```python
from build123d import *

# Parameters (mm, degrees)
BOSS_EXTRUDE1_DEPTH = 2.5
CUT_EXTRUDE1_DEPTH  = 10.5
FILLET1_R           = 0.25
CUT_EXTRUDE2_DEPTH  = 5.25
BOSS_EXTRUDE2_DEPTH = 0.5
CHAMFER1_SIZE       = 0.6
CHAMFER2_SIZE       = 0.4


with BuildPart() as part:
    # Sketch1 → Boss-Extrude1 (new body)
    with BuildSketch(Plane.XY):
        with BuildLine():
            Line((-2.75, -4), (-2.75, 4.05))
            ThreePointArc((-2.75, 4.05), (-2.544974747, 4.544974747), (-2.05, 4.75))
            Line((-2.05, 4.75), (2.05, 4.75))
            ThreePointArc((2.05, 4.75), (2.544974747, 4.544974747), (2.75, 4.05))
            Line((2.75, 4.05), (2.75, -4))
            Line((2.75, -4), (2.25, -4))
            Line((2.25, -4), (2.25, 4.05))
            ThreePointArc((2.25, 4.05), (2.191421356, 4.191421356), (2.05, 4.25))
            Line((2.05, 4.25), (-2.05, 4.25))
            ThreePointArc((-2.05, 4.25), (-2.191421356, 4.191421356), (-2.25, 4.05))
            Line((-2.25, 4.05), (-2.25, -4))
            Line((-2.25, -4), (-2.75, -4))
        make_face()
    extrude(amount=BOSS_EXTRUDE1_DEPTH)

    # Sketch2 → Cut-Extrude1 (cut)
    with BuildSketch(Plane(origin=(0, 4.75, 0), x_dir=(1, 0, 0), z_dir=(0, 1, 0))):
        with BuildLine():
            Line((-2.05, 0), (-1.725962279, -0.216025147))
            ThreePointArc((-1.725962279, -0.216025147), (-1.593504255, -0.278546013), (-1.448612181, -0.3))
            Line((-1.448612181, -0.3), (1.448612181, -0.3))
            ThreePointArc((1.448612181, -0.3), (1.593504255, -0.278546013), (1.725962279, -0.216025147))
            Line((1.725962279, -0.216025147), (2.05, 0))
            Line((2.05, 0), (2.05, 0.547519398))
            Line((2.05, 0.547519398), (-2.05, 0.547519398))
            Line((-2.05, 0.547519398), (-2.05, 0))
        make_face()
        with BuildLine():
            Line((-2.75, -2.5), (-2.345189488, -2.5))
            ThreePointArc((-2.345189488, -2.5), (-2.090994028, -2.430563198), (-1.907400646, -2.241538671))
            Line((-1.907400646, -2.241538671), (-1.321299677, -1.179230664))
            ThreePointArc((-1.321299677, -1.179230664), (-1.229502986, -1.084718401), (-1.102405256, -1.05))
            Line((-1.102405256, -1.05), (1.084290526, -1.05))
            ThreePointArc((1.084290526, -1.05), (1.222412736, -1.091619926), (1.314545856, -1.202621958))
            Line((1.314545856, -1.202621958), (1.734132573, -2.194756083))
            ThreePointArc((1.734132573, -2.194756083), (1.918398814, -2.416760148), (2.194643233, -2.5))
            Line((2.194643233, -2.5), (2.75, -2.5))
            Line((2.75, -2.5), (2.75, -3.056093585))
            Line((2.75, -3.056093585), (-2.75, -3.056093585))
            Line((-2.75, -3.056093585), (-2.75, -2.5))
        make_face()
    extrude(amount=-CUT_EXTRUDE1_DEPTH, mode=Mode.SUBTRACT)

    # Fillet1
    fillet1_edges = [part.edges().sort_by_distance(p)[0] for p in [
        (-2.05, 4.5, 0),
        (2.05, 4.5, 0),
    ]]
    fillet(fillet1_edges, radius=FILLET1_R)

    # Sketch3 → Cut-Extrude2 (cut, symmetric)
    with BuildSketch(Plane(origin=(0, 0, 0), x_dir=(0, 0, -1), z_dir=(1, 0, 0))):
        Polygon((0, 0.25), (-0.5, -0.35), (-0.5, -4.396314828), (0.876390697, -4.396314828), (0.876390697, 0.25), align=None)
        Polygon((-2.5, 0.25), (-2, -0.35), (-2, -4.896314828), (-3.070294312, -4.896314828), (-3.070294312, 0.25), align=None)
        with BuildLine():
            Line((-0.75, 3.024565065), (-0.75, 1.024565065))
            ThreePointArc((-0.75, 1.024565065), (-1.25, 0.524565065), (-1.75, 1.024565065))
            Line((-1.75, 1.024565065), (-1.75, 3.024565065))
            ThreePointArc((-1.75, 3.024565065), (-1.25, 3.524565065), (-0.75, 3.024565065))
        make_face()
    extrude(amount=CUT_EXTRUDE2_DEPTH, both=True, mode=Mode.SUBTRACT)

    # Sketch4 → Boss-Extrude2 (add, symmetric)
    with BuildSketch(Plane(origin=(0, 0, 0), x_dir=(0, 0, -1), z_dir=(1, 0, 0))):
        with BuildLine():
            Line((-1.05, 4.25), (-1.395169213, 3.954140675))
            ThreePointArc((-1.395169213, 3.954140675), (-1.770160684, 3.782160221), (-2.179373497, 3.834512432))
            Line((-2.179373497, 3.834512432), (-2.75, 4.079724782))
            Line((-2.75, 4.079724782), (-2.552592831, 4.539105245))
            Line((-2.552592831, 4.539105245), (-1.981966328, 4.293892895))
            ThreePointArc((-1.981966328, 4.293892895), (-1.845562057, 4.276442158), (-1.7205649, 4.333768976))
            Line((-1.7205649, 4.333768976), (-1.347308957, 4.653702641))
            ThreePointArc((-1.347308957, 4.653702641), (-1.225770907, 4.725154006), (-1.086992408, 4.75))
            Line((-1.086992408, 4.75), (-1.05, 4.75))
            Line((-1.05, 4.75), (-1.05, 4.25))
        make_face()
    extrude(amount=BOSS_EXTRUDE2_DEPTH, both=True)

    # Chamfer1
    chamfer1_edges = [part.edges().sort_by_distance(p)[0] for p in [
        (2.5, -4, 0.5),
        (-2.5, -4, 0.5),
    ]]
    chamfer(chamfer1_edges, length=CHAMFER1_SIZE)

    # Chamfer2
    chamfer2_edges = [part.edges().sort_by_distance(p)[0] for p in [
        (2.5, -4, 2),
        (-2.5, -4, 2),
    ]]
    chamfer(chamfer2_edges, length=CHAMFER2_SIZE)


solid = part.part
```
Input: part model. Units: mm. Frame: model coordinates. A direction names the side the tool comes from. Give positions to 0.01 mm unless a question says otherwise; leave off trailing zeros. Order: outer loops, then holes, each group sorted by start corner. A loop starts at its lowest first (then second) coordinate and runs counter-clockwise, first axis right, second up.
1. Set-up query: faces 5 (the face through (0, 4.75, 0.7)), 6 (the face through (0, 4.25, 0.7)), 7 (the face through (-0.5, 4, 2)), 8 (the face through (-2.25, 0, 1)). Return all of +Z, -Z, +X, -X, +Y, -Y with unobstructed straight access to the full face (end or side cutting, diameter ignored); none if empty.
Computed:
face 5: +Z, -Z, +X, -X, +Y
face 6: -Z, -Y
face 7: +Z, +Y, -Y
face 8: +Z, -Z, -Y
2. Cut plane B-B (y = -2.75). Return loops of the section in (x, z).
Computed:
outline: (-2.75, 0.5) - (-2.25, 0.5) - (-2.25, 2) - (-2.75, 2) - close; (2.25, 0.5) - (2.75, 0.5) - (2.75, 2) - (2.25, 2) - close
3. Line query: probe 1 along X at (y, z) = (-3, 0.85); probe 2 along Y at (x, z) = (-0.95, 0.85); probe 3 along Z at (x, y) = (2.5, -1.75). Output: solid intervals per line, ascending.
Computed:
probe 1: x = -2.75 to -2.25, 2.25 to 2.75
probe 2: y = 4.25 to 4.75
probe 3: z = 0.5 to 2
4. Cut plane C-C (x = 0.35). Return loops of the section in (y, z).
Computed:
outline: (3.83, 2.18) arc R0.75 ccw to (3.95, 1.4) - (4.25, 1.05) - (4.25, 0.3) - (4.75, 0.3) - (4.75, 1.09) arc R0.4 ccw to (4.65, 1.35) - (4.33, 1.72) arc R0.25 cw to (4.29, 1.98) - (4.54, 2.55) - (4.08, 2.75) - close
5. Cut plane A-A (y = 2.75). Return loops of the section in (x, z).
Computed:
outline: (-2.75, 0) - (-2.25, 0) - (-2.25, 0.75) - (-2.75, 0.75) - close; (-2.75, 1.75) - (-2.25, 1.75) - (-2.25, 2.49) arc R0.5 ccw to (-2.35, 2.5) - (-2.75, 2.5) - close; (2.25, 0) - (2.75, 0) - (2.75, 0.75) - (2.25, 0.75) - close; (2.25, 1.75) - (2.75, 1.75) - (2.75, 2.5) - (2.25, 2.5) - close
6. Draft query along X for faces 1 (the face through (2.25, 0, 1)), 2 (the face through (-2.75, 0, 1)), 3 (the face through (0.5, 4, 2)), 4 (the face through (2.75, 0, 1)). Return one class per face: released by +X, released by -X, zero draft, split by the parting line, or undercut.
Computed:
face 1: undercut
face 2: released by -X
face 3: undercut
face 4: released by +X
7. Pin query (flat end, axial travel): pin 1 Ø1 at (x, y) = (0, -1.5) entering from +Z; pin 2 Ø0.6 at (x, y) = (0, 4.5) entering from -Z; pin 3 Ø0.6 at (x, y) = (-2.5, -1.5) entering from -Z. Return the tip coordinate at first contact, or that it passes through.
Computed:
pin 1: passes through
pin 2: stops at z = 0.3
pin 3: stops at z = 0.5
